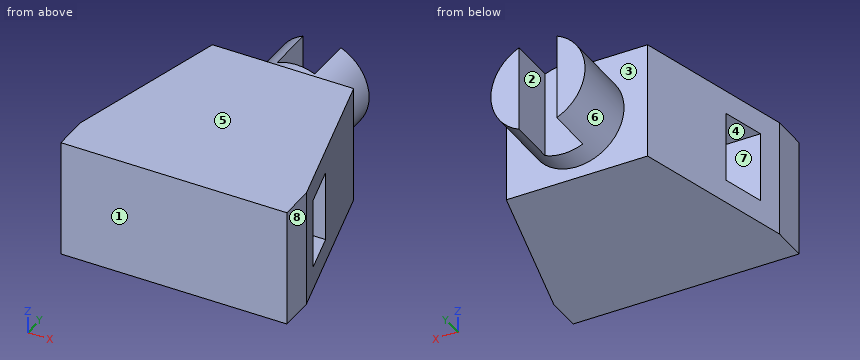
from build123d import *

# Parameters (mm, degrees)
SKETCH1_W           = 96
SKETCH1_H           = 50
BOSS_EXTRUDE1_DEPTH = 84
SKETCH5_W           = 30
SKETCH5_H           = 18
CUT_EXTRUDE2_DEPTH  = 102
CUT_EXTRUDE1_START  = -51
CUT_EXTRUDE1_DEPTH  = 52
SKETCH6_R           = 20
BOSS_EXTRUDE2_DEPTH = 30
CUT_EXTRUDE3_DEPTH  = 20


with BuildPart() as part:
    # Sketch1 → Boss-Extrude1 (new body)
    with BuildSketch(Plane(origin=(0, 0, 0), x_dir=(1, 0, 0), z_dir=(0, 1, 0))):
        with Locations((48, 25)):
            Rectangle(SKETCH1_W, SKETCH1_H)
    extrude(amount=BOSS_EXTRUDE1_DEPTH)

    # Sketch5 → Cut-Extrude2 (cut)
    with BuildSketch(Plane.ZY):
        with Locations((-25, 34)):
            Rectangle(SKETCH5_W, SKETCH5_H)
    extrude(amount=-CUT_EXTRUDE2_DEPTH, mode=Mode.SUBTRACT)

    # Sketch2 → Cut-Extrude1 (cut)
    with BuildSketch(Plane.XY.offset(CUT_EXTRUDE1_START)):
        Polygon((-62.209054952, -223.468043983), (0, 15), (18, 84), (80.209054952, 322.468043983), (-396.727033013, 446.886153886), (-539.145142917, -99.049934079), align=None)
    cut_extrude1 = extrude(amount=CUT_EXTRUDE1_DEPTH, mode=Mode.SUBTRACT)

    # Mirror1: Cut-Extrude1 across plane
    add(cut_extrude1.mirror(Plane.ZY.offset(-48)), mode=Mode.SUBTRACT)

    # Sketch6 → Boss-Extrude2 (add)
    with BuildSketch(Plane(origin=(0, 84, 0), x_dir=(1, 0, 0), z_dir=(0, 1, 0))):
        with Locations((48, 25)):
            Circle(SKETCH6_R)
    extrude(amount=BOSS_EXTRUDE2_DEPTH)

    # Sketch8 → Cut-Extrude3 (cut)
    with BuildSketch(Plane(origin=(0, 114, 0), x_dir=(1, 0, 0), z_dir=(0, 1, 0))):
        with BuildLine():
            Line((40, 6.66969722), (40, 43.33030278))
            ThreePointArc((40, 43.33030278), (48, 45), (56, 43.33030278))
            Line((56, 43.33030278), (56, 6.66969722))
            ThreePointArc((56, 6.66969722), (48, 5), (40, 6.66969722))
        make_face()
    extrude(amount=-CUT_EXTRUDE3_DEPTH, mode=Mode.SUBTRACT)


solid = part.part
Check sheet for the modelled part. Datum: model origin and axes. Units: mm. Face numbers are marked on the shaded views. A direction names the side the tool comes from. Round coordinates to 2 decimals unless told otherwise and drop trailing zeros. Loops run counter-clockwise (first coordinate to the right, second up) from the corner with the lowest first, then second, coordinate; pieces in that order, holes last. Notation, with made-up numbers: M -7,5.25 L 40,5.25 A23 cw 40,13.25 Z; hole C 43,-10 d11. An arc over 180 degrees is marked long. One line per item, written item: value.
(1) Sectioned sample at D-D, the plane x = 60. Record the cut outline in (y, z), then the cut area to 3 significant figures.
Computed values:
outline: M 0,-50 L 84,-50 L 84,-41 L 114,-41 L 114,-9 L 84,-9 L 84,0 L 0,0 Z; hole M 25,-40 L 43,-40 L 43,-10 L 25,-10 Z
area: 4,620 mm^2
(2) Sectioned sample at C-C, the plane y = 37. Record the cut outline in (x, z).
Computed values:
outline: M 5.74,-50 L 90.26,-50 L 90.26,-40 L 5.74,-40 Z; M 5.74,-10 L 90.26,-10 L 90.26,0 L 5.74,0 Z
(3) Thickness scan on line 1 (Y direction, x = 59, z = -26); line 2 (Z direction, x = 39.5, y = 26); line 3 (Y direction, x = 23, z = -36.5). Record the ranges inside material, lowest first.
Computed values:
line 1: y = 0 to 25, 43 to 114
line 2: z = -50 to -40, -10 to 0
line 3: y = 0 to 25, 43 to 84
(4) Depth check by flat-ended pin: pin 1 Ø12 at (y, z) = (60, -26) entering from +X; pin 2 Ø1.5 at (y, z) = (48.5, -24.5) entering from +X; pin 3 Ø1.5 at (y, z) = (16.5, -7) entering from -X. Enter the tip coordinate at first touch or a pass-through.
Computed values:
pin 1: stops at x = 85.83
pin 2: stops at x = 87.46
pin 3: stops at x = 0.2
(5) Release check for a two-part mould opening along Z. For the marked faces 6, 7 and 8 record: +Z half, -Z half, draft (parallel to the pull), parting line (faces both ways), or undercut.
Computed values:
face 6: parting line
face 7: undercut
face 8: draft
(6) Access from +Z, -Z, +X, -X, +Y, -Y to the whole of each face (thin tool, end or side, straight path). Record for the marked faces 1, 2, 3, 4 and 5.
Computed values:
face 1: +Z, -Z, +X, -X, -Y
face 2: +Z, -Z, +Y
face 3: +Y
face 4: +X, -X
face 5: +Z, +X, -X, +Y, -Y
(7) Sectioned sample at A-A, the plane x = 25. Record the cut outline in (y, z).
Computed values:
outline: M 0,-50 L 84,-50 L 84,0 L 0,0 Z; hole M 25,-40 L 43,-40 L 43,-10 L 25,-10 Z
(8) Sectioned sample at B-B, the plane z = -25. Record the cut outline in (x, y).
Computed values:
outline: M 0,0 L 96,0 L 96,15 L 93.39,25 L 2.61,25 L 0,15 Z; M 7.3,43 L 88.7,43 L 78,84 L 68,84 L 68,114 L 56,114 L 56,94 L 40,94 L 40,114 L 28,114 L 28,84 L 18,84 Z
